Here's how the part is built. I have some questions about the finished solid (model axes, mm). A direction names the side the tool comes from. Give positions to 0.01 mm unless a question says otherwise; leave off trailing zeros. Order: outer loops, then holes, each group sorted by start corner. A loop starts at its lowest first (then second) coordinate and runs counter-clockwise, first axis right, second up. Notation, with made-up numbers: (63, -35) - (100, -35) arc R19 cw to (100, -21) - close; hole circle Ø10 at (-23.75, -6.5). An arc over 180 degrees is marked (long way). One line per question, with ' | ' between items.
from build123d import *

# Parameters (mm, degrees)
BOSS_EXTRUDE2_DEPTH = 49.3
SKETCH3_R           = 1
CUT_EXTRUDE1_DEPTH  = 55.974100913
SKETCH4_R           = 2.25
CUT_EXTRUDE2_DEPTH  = 56.188642368
SKETCH5_W           = 25
SKETCH5_H           = 8
CUT_EXTRUDE3_DEPTH  = 55.974100913
FILLET1_R           = 2


with BuildPart() as part:
    # Sketch2 → Boss-Extrude2 (new body)
    with BuildSketch(Plane.XY):
        with BuildLine():
            Line((-2.241180955, -1.965925826), (-11.900439218, -4.554116277))
            Line((-11.900439218, -4.554116277), (-11.123982082, -7.451893756))
            Line((-11.123982082, -7.451893756), (-1.46472382, -4.863703305))
            ThreePointArc((-1.46472382, -4.863703305), (0.673413361, -3.435045716), (1.5, -1))
            Line((1.5, -1), (1.5, 20.3))
            Line((1.5, 20.3), (-1.5, 20.3))
            Line((-1.5, 20.3), (-1.5, -1))
            ThreePointArc((-1.5, -1), (-1.70664666, -1.608761429), (-2.241180955, -1.965925826))
        make_face()
    extrude(amount=BOSS_EXTRUDE2_DEPTH)

    # Sketch3 → Cut-Extrude1 (cut, through all)
    with BuildSketch(Plane(origin=(1.5, 0, 0), x_dir=(0, 0, -1), z_dir=(1, 0, 0))):
        with Locations(Location((-45.3, 17.8, 0), (0, 0, 90))):
            Circle(SKETCH3_R)
        with Locations(Location((-4, 17.8, 0), (0, 0, 90))):
            Circle(SKETCH3_R)
        with Locations(Location((-4, 1.5, 0), (0, 0, 90))):
            Circle(SKETCH3_R)
        with Locations(Location((-45.3, 1.5, 0), (0, 0, 90))):
            Circle(SKETCH3_R)
    extrude(amount=-CUT_EXTRUDE1_DEPTH, mode=Mode.SUBTRACT)

    # Sketch4 → Cut-Extrude2 (cut, through all)
    with BuildSketch(Plane(origin=(0.3413508, -1.273938528, 0), x_dir=(0.96592582628907, 0.25881904510251463, 0), z_dir=(-0.25881904510251463, 0.96592582628907, 0))):
        with Locations(Location((-7.673633611, -8, 0), (0, 0, 180))):
            Circle(SKETCH4_R)
        with Locations(Location((-7.673633611, -41.3, 0), (0, 0, 180))):
            Circle(SKETCH4_R)
    extrude(amount=-CUT_EXTRUDE2_DEPTH, mode=Mode.SUBTRACT)

    # Sketch5 → Cut-Extrude3 (cut, through all)
    with BuildSketch(Plane(origin=(1.5, 0, 0), x_dir=(0, 0, -1), z_dir=(1, 0, 0))):
        with Locations((-24.65, 16.3)):
            Rectangle(SKETCH5_W, SKETCH5_H)
    extrude(amount=-CUT_EXTRUDE3_DEPTH, mode=Mode.SUBTRACT)

    # Fillet1
    fillet1_edges = [part.edges().sort_by_distance(p)[0] for p in [
        (0, 20.3, 12.15),
        (0, 20.3, 37.15),
        (0, 12.3, 12.15),
        (0, 12.3, 37.15),
    ]]
    fillet(fillet1_edges, radius=FILLET1_R)


solid = part.part
1) On a 3-axis mill with a long thin cutter (end or side, diameter ignored), from which of +Z, -Z, +X, -X, +Y, -Y can I reach the whole of each face in a straight line? I mean faces 4 (the face through (0.02, 1.37, 4.99)), 5 (the face through (-0.02, 19.73, 11.55)). Say none if no direction works.
Model answer:
face 4: +X, -X | face 5: +X, -X, +Y
2) I want a section at C-C (z = 4). List the corners of the cut face in (x, y) for me.
Model answer:
outline: (-11.9, -4.55) - (-11.12, -7.45) - (-1.46, -4.86) arc R4 ccw to (1.5, -1) - (1.5, 0.5) - (-1.5, 0.5) - (-1.5, -1) arc R1 cw to (-2.24, -1.97) - close; (-1.5, 2.5) - (1.5, 2.5) - (1.5, 16.8) - (-1.5, 16.8) - close; (-1.5, 18.8) - (1.5, 18.8) - (1.5, 20.3) - (-1.5, 20.3) - close
3) I want a section at B-B (y = 1.5). List the corners of the cut face in (x, z) for me, plus the area to 3 significant figures.
Model answer:
outline: (-1.5, 0) - (1.5, 0) - (1.5, 3) - (-1.5, 3) - close; (-1.5, 5) - (1.5, 5) - (1.5, 44.3) - (-1.5, 44.3) - close; (-1.5, 46.3) - (1.5, 46.3) - (1.5, 49.3) - (-1.5, 49.3) - close | area: 136 mm2
4) Thinking about a two-plate mould opening in Z: for faces 1 (the face through (-1.5, 7, 24)), 2 (the face through (-1, 4, 49.3)), 3 (the face through (0, 16, 12.15)), which applies, +Z half, -Z half, draft (parallel to the pull), parting line (faces both ways), or undercut?
Model answer:
face 1: draft | face 2: +Z half | face 3: undercut
5) Please list where these lines run through material, in increasing order: L1, parallel to Z at x = 0.1, y = 1.5; L2, parallel to Z at x = 0.75, y = 16.75; L3, parallel to X at y = 13.5, z = 41.
Model answer:
L1: z = 0 to 3, 5 to 44.3, 46.3 to 49.3 | L2: z = 0 to 12.15, 37.15 to 49.3 | L3: x = -1.5 to 1.5
6) I want a section at D-D (z = 22). List the corners of the cut face in (x, y) for me, plus the area to 3 significant figures.
Model answer:
outline: (-11.9, -4.55) - (-11.12, -7.45) - (-1.46, -4.86) arc R4 ccw to (1.5, -1) - (1.5, 12.3) - (-1.5, 12.3) - (-1.5, -1) arc R1 cw to (-2.24, -1.97) - close | area: 79.7 mm2
7) I want a section at A-A (y = 17.8). List the corners of the cut face in (x, z) for me.
Model answer:
outline: (-1.5, 0) - (1.5, 0) - (1.5, 3) - (-1.5, 3) - close; (-1.5, 5) - (1.5, 5) - (1.5, 12.15) - (-1.5, 12.15) - close; (-1.5, 37.15) - (1.5, 37.15) - (1.5, 44.3) - (-1.5, 44.3) - close; (-1.5, 46.3) - (1.5, 46.3) - (1.5, 49.3) - (-1.5, 49.3) - close
8) I'm going to push flat-ended pins straight in: P1, Ø1.5, axis at x = -8.5, z = 6, coming from the +Y side; P2, Ø6.5, axis at y = 10.5, z = 34, coming from the -X side; P3, Ø8, axis at x = -1.5, z = 42, coming from the -Y side; P4, Ø8, axis at x = -7.5, y = 1.5, coming from the -Z side. Where does each tip first touch, or does it pass through?
Model answer:
P1: stops at y = -3.45 | P2: stops at x = -1.5 | P3: stops at y = -5.89 | P4: passes through
